Part model, mm, in its own coordinate system. Coordinates: 2 decimals unless noted, no trailing zeros. Loops run counter-clockwise (first coordinate to the right, second up) from the corner with the lowest first, then second, coordinate; pieces in that order, holes last. Notation, with made-up numbers: (15.5, 36.25) -> (57.5, 36.25) arc R36 ccw to (57.5, 70.25) -> close; hole circle Ø6 at (36, -36). An arc over 180 degrees is marked (long way). One line per question, with ' | ' between items. Start each with the question number.
1) Drop flat-ended pins along their axis: pin 1 (10 mm diameter, centred on x = 5, z = -8.5, fed in from -Y); pin 2 (11 mm diameter, centred on x = 3, z = -6, fed in from +Y); pin 3 (12 mm diameter, centred on x = 8, z = -9, fed in from +Y); pin 4 (3 mm diameter, centred on y = 2, z = -10, fed in from +X). Give the stop position or say it passes through.
2) Cut at C-C (z = -10). List the corners of the cut face in (x, y).
3) Probe L1, parallel to Z at x = 0, y = -11; L2, parallel to Y at x = -3, z = 6; L3, parallel to Z at x = 7, y = -9. List the from-to ranges inside material, lowest first. Write a range as from..to.
4) Two-plate mould, pull along Z, no slides. Class faces 1 (the face through (0.585, 6.409, -2.636)), 2 (the face through (0, 15, 0)), 3 (the face through (-2.018, -10.395, 15.368)), 4 (the face through (0, -3, 0)): released by +Z, released by -Z, zero draft, split by the parting line, or undercut.
5) Cut at D-D (y = 7). List the corners of the cut face in (x, z), plus the area to 3 significant figures.
6) Cut at B-B (x = -8.5). List the corners of the cut face in (y, z).
7) Cut at A-A (y = -15). List the corners of the cut face in (x, z), plus the area to 3 significant figures.
from build123d import *

# Parameters (mm, degrees)
F0_R     = 18.5
F1_DEPTH = 18
F2_T     = -3
F3_R     = 2.7
F4_DEPTH = 15
F5_R     = 2


with BuildPart() as f1:
    # F0 (on Front) → F1 (new body)
    with BuildSketch(Plane.XZ):
        Circle(F0_R)
    extrude(amount=F1_DEPTH)

    # F2
    f2_openings = [f1.faces().sort_by_distance(p)[0] for p in [
        (0, -18, 0),
    ]]
    offset(amount=F2_T, openings=f2_openings)

    # F3 (on face) → F4 (join)
    with BuildSketch(Plane(origin=(0, 0, 0), x_dir=(-1, 0, 0), z_dir=(0, 1, 0))):
        Circle(F3_R)
    extrude(amount=F4_DEPTH)

    # F5
    f5_edges = [f1.edges().sort_by_distance(p)[0] for p in [
        (2.7, 15, 0),
    ]]
    fillet(f5_edges, radius=F5_R)


solid = f1.part
Reported:
1) pin 1: stops at y = -3 | pin 2: stops at y = 14.93 | pin 3: stops at y = 0 | pin 4: passes through
2) outline: (-15.56, -18) -> (-11.84, -18) -> (-11.84, -3) -> (11.84, -3) -> (11.84, -18) -> (15.56, -18) -> (15.56, 0) -> (-15.56, 0) -> close
3) L1: z = -18.5..-15.5, 15.5..18.5 | L2: y = -3..0 | L3: z = -17.12..-13.83, 13.83..17.12
4) face 1: split by the parting line | face 2: zero draft | face 3: undercut | face 4: undercut
5) outline: circle Ø5.4 at (0, 0) | area: 22.9 mm²
6) outline: (-18, -16.43) -> (0, -16.43) -> (0, 16.43) -> (-18, 16.43) -> (-18, 12.96) -> (-3, 12.96) -> (-3, -12.96) -> (-18, -12.96) -> close
7) outline: circle Ø37 at (0, 0); hole circle Ø31 at (0, 0) | area: 320 mm²
